Work out the finished part from the listing and answer in its coordinate system (mm). A direction names the side the tool comes from. Coordinates: 2 decimals unless noted, no trailing zeros. Order: outer loops, then holes, each group sorted by start corner. A loop starts at its lowest first (then second) coordinate and runs counter-clockwise, first axis right, second up. Notation, with made-up numbers: (45, -34) - (76, -34) arc R25 ccw to (76, -18) - close; hole circle Ø2 at (-21.5, 80.25). An arc over 180 degrees is marked (long way). Answer as a JSON object with one key per item and string values. Group by question number.
1) Section A-A (y = 10) is taken. Give the vertices of the cut face in (x, z).
2) Section C-C (z = -5.75) is taken. Give the vertices of the cut face in (x, y), plus the area to 3 significant figures.
3) Find the intervals of material crossed by line 1 along Y through (x, z) = (-1.75, 4.75); line 2 along X through (y, z) = (23, -2); line 3 along Y through (x, z) = (-2.75, -0.25), in increasing order.
4) Section B-B (z = 5.5) is taken. Give the vertices of the cut face in (x, y).
5) A tool of negligible diameter and unlimited length cuts with its end or side. For faces 4 (the face through (-2.34, 26.117, -3.55)), 5 (the face through (0.96, 27.37, 4.34)), 6 (the face through (-1.9, 26.117, 3.8)), 7 (the face through (1.83, 26.117, -3.81)), 8 (the face through (2.26, 16.24, 3.38)), from which of +Z, -Z, +X, -X, +Y, -Y can it reach the whole face along a straight path? Write none if from no direction.
6) The mould has two halves that part along Y. Classify faces 1 (the face through (0, 0, 0)), 2 (the face through (8, 3.1, 2.5)), 3 (the face through (-2.26, 16.24, -3.38)): released by +Y, released by -Y, zero draft, split by the parting line, or undercut.
7) Each of these flat-tipped pins is pushed along its axis until it touches: P1, Ø7, axis at x = 1, z = -1.5, coming from the +Y side; P2, Ø1, axis at x = -3.5, z = -2, coming from the +Y side; P3, Ø6, axis at x = 5, z = -4, coming from the +Y side; P4, Ø4, axis at y = 20.5, z = -1.5, coming from the -X side. Where does it stop, or does it pass through?
from build123d import *

# Parameters (mm, degrees)
F3_DEPTH = 26.416
F2_R     = 8.382
F4_DEPTH = 6.35


with BuildPart() as f1:
    # F0 (on Top) → F1 (revolve)
    with BuildSketch(Plane.XY):
        with BuildLine():
            Line((0, 28.657248), (0, 37.445775))
            ThreePointArc((0, 37.445775), (-4.419559, 33.475669), (-0.944353, 28.657248))
            Line((-0.944353, 28.657248), (-4.445, 28.657248))
            Line((-4.445, 28.657248), (-4.445, 26.117248))
            Line((-4.445, 26.117248), (0, 26.117248))
            Line((0, 26.117248), (0, 28.555775))
            Line((0, 28.555775), (0, 28.657248))
        make_face()
    revolve(axis=Axis((0, 33.000775, 0), (0, -1, 0)))

    # F2 (on Front) → F3 (join)
    with BuildSketch(Plane.XZ):
        Polygon((-4.192043, -2.109085), (-0.269501, -4.684958), (3.922542, -2.575873), (4.192043, 2.109085), (0.269501, 4.684958), (-3.922542, 2.575873), align=None)
    extrude(amount=-F3_DEPTH)

    # F2 (on Front) → F4 (join)
    with BuildSketch(Plane.XZ):
        Circle(F2_R)
        Polygon((3.922542, -2.575873), (-0.269501, -4.684958), (-4.192043, -2.109085), (-3.922542, 2.575873), (0.269501, 4.684958), (4.192043, 2.109085), align=None, mode=Mode.SUBTRACT)
    extrude(amount=-F4_DEPTH)


solid = f1.part
Report:
{
 "1": {"outline": "(-4.19, -2.11) - (-0.27, -4.68) - (3.92, -2.58) - (4.19, 2.11) - (0.27, 4.68) - (-3.92, 2.58) - close"},
 "2": {"outline": "(-6.1, 0) - (6.1, 0) - (6.1, 6.35) - (-6.1, 6.35) - close", "area": "77.5 mm²"},
 "3": {"line 1": "y = 0 to 6.35", "line 2": "x = -4.19 to 3.96", "line 3": "y = 0 to 28.66, 29.52 to 36.48"},
 "4": {"outline": "(-6.33, 0) - (6.33, 0) - (6.33, 6.35) - (-6.33, 6.35) - close"},
 "5": {"face 4": "-Z, -X", "face 5": "+Y", "face 6": "+Z, -X", "face 7": "-Z, +X", "face 8": "+Z, +X"},
 "6": {"face 1": "released by -Y", "face 2": "zero draft", "face 3": "undercut"},
 "7": {"P1": "stops at y = 37.45", "P2": "stops at y = 35.7", "P3": "stops at y = 35.86", "P4": "stops at x = -4.19"}
}
